Build history of the part. All positions in model axes, mm. A direction names the side the tool comes from. Coordinates: 2 decimals unless noted, no trailing zeros. Write each loop counter-clockwise with the first axis right and the second up, starting at its lowest first coordinate (ties: lowest second). Pieces come first, ordered by that corner, then holes. Notation, with made-up numbers: (85.5, 57.5) -> (143.5, 57.5) arc R12 ccw to (143.5, 74.5) -> close; hole circle Ø8 at (-17, 82). An arc over 180 degrees is marked (long way). Write each question's results on one line, items separated by ' | '. Start each with the question number.
Q1. Tool access for faces 4 (the face through (1.972, 40.476, 87.688)), 5 (the face through (0, 97, 30)), 6 (the face through (1.97, 65.69, 70.85)): list every direction of +Z, -Z, +X, -X, +Y, -Y with a clear straight run to the whole face (end or side of a thin tool).
Q2. Drop flat-ended pins along their axis: pin 1 Ø1.5 at (x, y) = (1.5, 204) entering from +Z; pin 2 Ø2 at (x, z) = (2.5, 17) entering from -Y; pin 3 Ø2 at (x, y) = (2, 192) entering from -Z. Give the stop position or say it passes through.
Q3. Saw through at C-C on z = 53. Give the cut face in (x, y).
Q4. Saw through at B-B on y = 235. Give the cut face in (x, z), and give its area (3 significant figures).
Q5. Two-plate mould, pull along Y, no slides. Class faces 1 (the face through (1.97, 182.79, 30.06)), 2 (the face through (4, 97, 30)), 3 (the face through (1.97, 218.18, 25.78)): released by +Y, released by -Y, zero draft, split by the parting line, or undercut.
Q6. Drill centre lines: line 1 (Z direction, x = 2.7, y = 58); line 2 (Z direction, x = 2.4, y = 215.5); line 3 (Y direction, x = 3.5, z = 100). Where is each one in solid material? Low to high.
Autodesk Fusion 360 part; units mm, degrees
sketch "スケッチ1" plane through (0, 0, 0) normal (1, 0, 0) x (0, 0, -1)
  line L0 (-116, 0) -> (-116, 20)
  line L1 (-116, 20) -> (-111.3943, 33.2207)
  line L2 (-111.3943, 33.2207) -> (-101.951, 29.931)
  line L3 (-101.951, 29.931) -> (-105.2407, 20.4876)
  line L4 (-105.2407, 20.4876) -> (-95.7973, 17.1978)
  line L5 (-14, 252) -> (0, 252)
  line L6 (-95.7973, 17.1978) -> (-79.3485, 64.4147)
  line L7 (-79.3485, 64.4147) -> (-65.1834, 59.4801)
  line L8 (-65.1834, 59.4801) -> (-63.8675, 63.2574)
  line L9 (-63.8675, 63.2574) -> (-78.0326, 68.1921)
  line L10 (-78.0326, 68.1921) -> (-38.5555, 181.5127)
  line L11 (-38.5555, 181.5127) -> (-24.3904, 176.578)
  line L12 (-24.3904, 176.578) -> (-23.0745, 180.3554)
  line L13 (-23.0745, 180.3554) -> (-37.2396, 185.29)
  line L14 (-37.2396, 185.29) -> (-14, 252)
  line L15 (-116, 0) -> (-70, 0)
  line L16 (-70, 0) -> (-70, -4)
  line L17 (-70, -4) -> (-50, -4)
  line L18 (-50, -4) -> (-50, 0)
  line L19 (-50, 0) -> (0, 0)
  line L20 (0, 252) -> (0, 165)
  line L21 (0, 165) -> (4, 165)
  line L22 (4, 165) -> (4, 145)
  line L23 (4, 145) -> (0, 145)
  line L24 (0, 145) -> (0, 0)
  line L25 (4, 155) -> (-13.5, 155)
  line L26 (-60, -4) -> (-60, 13.5)
  line L27 (-64.1481, 77.6509) -> (-33.5533, 165.4743)
  line L28 (-10, 10) -> (-30, 10)
  line L29 (-30, 10) -> (-30, 30)
  line L30 (-30, 30) -> (-10, 30)
  line L31 (-10, 30) -> (-10, 10)
  dimension "d1" = 116
  dimension "d2" = 20
  dimension "d3" = 14
  dimension "d4" = 10
  dimension "d5" = 10
  dimension "d6" = 10
  dimension "d9" = 14
  dimension "d11" = 252
  dimension "d12" = 248.642
  dimension "d13" = 4
  dimension "d14" = 4
  dimension "d15" = 120
  dimension "d16" = 50
  dimension "d17" = 15
  dimension "d18" = 20
  dimension "d19" = 4
  dimension "d20" = 50
  dimension "d21" = 4
  dimension "d22" = 20
  dimension "d23" = 145
  dimension "d24" = 17.5
  dimension "d25" = 17.5
  dimension "d31" = 10
  dimension "d32" = 13.5
  dimension "d33" = 13.5
  dimension "d36" = 10
  dimension "d37" = 20
  dimension "d38" = 20
  dimension "d39" = 10
extrude "押し出し1" add sketch "スケッチ1" along normal blind 4
hole "穴1" at (0, 0, 0) at (0, 13.5, 60) at (0, 0, 0) at (0, 165.4743, 33.5533) direction (-1, 0, 0) diameter 3.2 end through all
fillet "フィレット1" radius 1 2 edges at (2, 29.931, 101.951) (2, 33.2207, 111.3943)
Returned:
1) face 4: +X, -X, +Y | face 5: +Z, -Z, -X, +Y, -Y | face 6: +X, -X
2) pin 1: stops at z = 30.98 | pin 2: stops at y = 0 | pin 3: stops at z = 0
3) outline: (0, -4) -> (4, -4) -> (4, 140.05) -> (0, 140.05) -> close
4) outline: (0, 0) -> (4, 0) -> (4, 19.92) -> (0, 19.92) -> close | area: 79.7 mm2
5) face 1: undercut | face 2: zero draft | face 3: released by +Y
6) line 1: z = 0 to 81.58 | line 2: z = 0 to 26.72 | line 3: y = 0 to 18.66
